Geometry check sheet. Reference: drawing and pictorial views, mm from the part's lowest x, y, z. A direction names the side the tool comes from. Coordinates: 2 decimals unless noted, no trailing zeros. Loops run counter-clockwise (first coordinate to the right, second up) from the corner with the lowest first, then second, coordinate; pieces in that order, holes last. Notation, with made-up numbers: (88.25, -20.5) -> (121.25, -20.5) arc R21 ccw to (121.25, -15.5) -> close; hole circle Ø1 at (29, 52). An arc over 180 degrees is marked (long way). Answer as a JSON object with one key per item and string values. Group by question number.
Q1. Set-up check for the marked faces 1, 2 and 3: record each of +Z, -Z, +X, -X, +Y, -Y from which the full face is reachable in a straight line by a thin tool's end or side.
Q2. Scan lines: L1, parallel to Y at x = 3, z = 0.4; L2, parallel to Y at x = 11.25, z = 4.3; L3, parallel to X at y = 35.5, z = 3.2. Record each from-to range of solid material in increasing order.
Q3. Cross-section at B-B on z = 2.7. Record the boundary of the cut face in (x, y), and give its area (3 significant figures).
Q4. Cross-section at A-A on x = 13.5. Record the boundary of the cut face in (y, z), and give its area (3 significant figures).
Q5. Gauge pin test, flat ends, axial feed: pin 1 Ø3 at (x, z) = (7.5, 3) entering from -Y; pin 2 Ø1.2 at (x, y) = (7.5, 35) entering from +Z; pin 3 Ø0.9 at (y, z) = (36, 2.5) entering from -X. Record the tip position at first contact, or that the pin passes through.
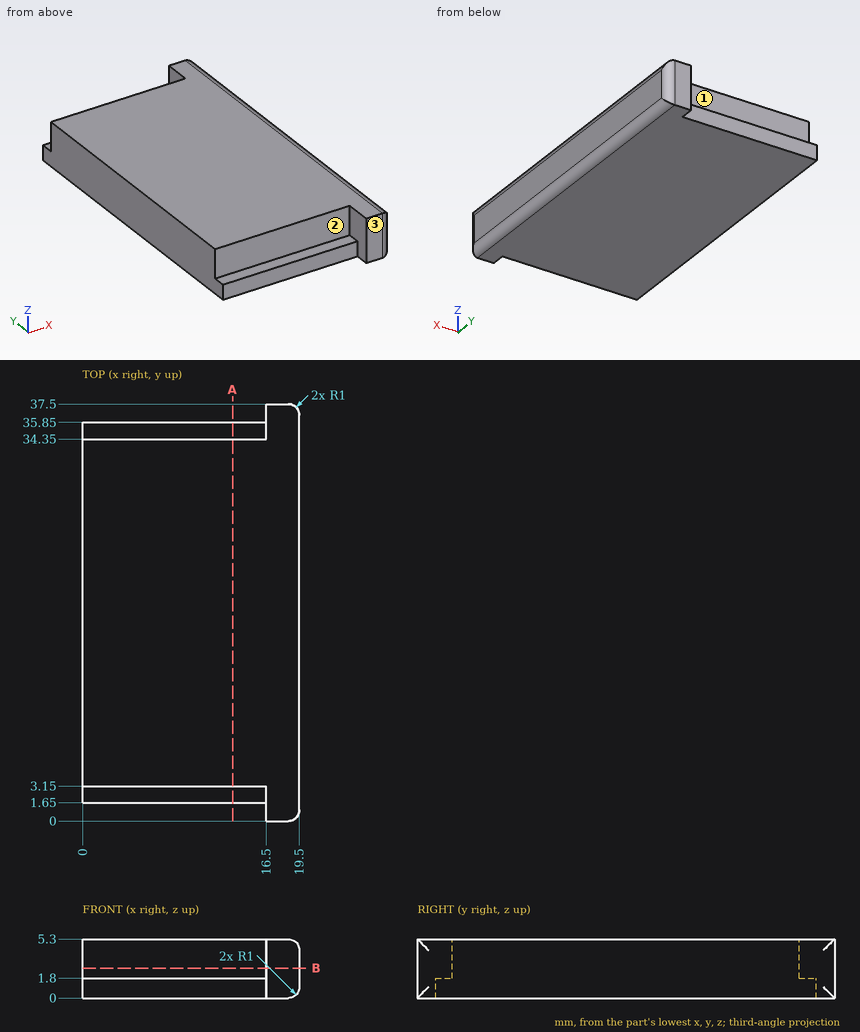
Computed values:
{
 "1": {"face 1": "+Z, -X, +Y", "face 2": "+Z, -X, -Y", "face 3": "+Z, -Z, +X, -X, -Y"},
 "2": {"L1": "y = 1.65 to 35.85", "L2": "y = 3.15 to 34.35", "L3": "x = 16.5 to 19.5"},
 "3": {"outline": "(0, 3.15) -> (16.5, 3.15) -> (16.5, 0) -> (18.5, 0) arc R1 ccw to (19.5, 1) -> (19.5, 36.5) arc R1 ccw to (18.5, 37.5) -> (16.5, 37.5) -> (16.5, 34.35) -> (0, 34.35) -> close", "area": "627 mm²"},
 "4": {"outline": "(1.65, 0) -> (35.85, 0) -> (35.85, 1.8) -> (34.35, 1.8) -> (34.35, 5.3) -> (3.15, 5.3) -> (3.15, 1.8) -> (1.65, 1.8) -> close", "area": "171 mm²"},
 "5": {"pin 1": "stops at y = 1.65", "pin 2": "stops at z = 1.8", "pin 3": "stops at x = 16.5"}
}
